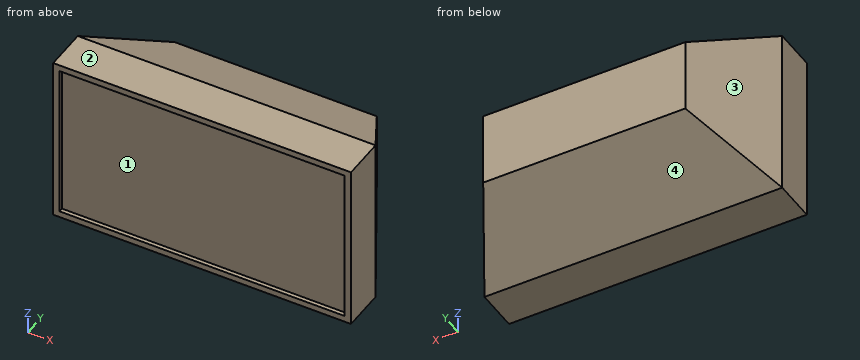
from build123d import *

# Parameters (mm, degrees)
F0_W        = 140
F0_H        = 80
F1_DEPTH    = 60
F2_C1_SIZE2 = 22.5
F2_C1_SIZE  = 40
F2_C2_SIZE2 = 22.5
F2_C2_SIZE  = 40
F2_C3_SIZE2 = 40
F2_C3_SIZE  = 22.5
F2_C4_SIZE2 = 40
F2_C4_SIZE  = 22.5
F3_W        = 134
F3_H        = 74
F4_DEPTH    = 2
F5_DEPTH    = 2


with BuildPart() as f1:
    # F0 (on Front) → F1 (new body)
    with BuildSketch(Plane.XZ):
        Rectangle(F0_W, F0_H)
    extrude(amount=F1_DEPTH)

    # F2: chamfer of 22.5 x 40 on 4 edges, made by hand

    # F2_c1
    f2_c1_edges = [f1.edges().sort_by_distance(p)[0] for p in [
        (0, 0, -40),
    ]]
    f2_c1_side = f1.faces().sort_by_distance((0, -0.45, -40))[0]
    chamfer(f2_c1_edges, length=F2_C1_SIZE, length2=F2_C1_SIZE2, reference=f2_c1_side)

    # F2_c2
    f2_c2_edges = [f1.edges().sort_by_distance(p)[0] for p in [
        (70, 0, 11.25),
    ]]
    f2_c2_side = f1.faces().sort_by_distance((70, -0.45, 11.25))[0]
    chamfer(f2_c2_edges, length=F2_C2_SIZE, length2=F2_C2_SIZE2, reference=f2_c2_side)

    # F2_c3
    f2_c3_edges = [f1.edges().sort_by_distance(p)[0] for p in [
        (-11.25, 0, 40),
    ]]
    f2_c3_side = f1.faces().sort_by_distance((-11.25, 0, 39.55))[0]
    chamfer(f2_c3_edges, length=F2_C3_SIZE, length2=F2_C3_SIZE2, reference=f2_c3_side)

    # F2_c4
    f2_c4_edges = [f1.edges().sort_by_distance(p)[0] for p in [
        (-70, 0, 0),
    ]]
    f2_c4_side = f1.faces().sort_by_distance((-69.55, 0, 0))[0]
    chamfer(f2_c4_edges, length=F2_C4_SIZE, length2=F2_C4_SIZE2, reference=f2_c4_side)

    # F3 (on face) → F4 (join)
    with BuildSketch(Plane.XZ.offset(60)):
        Rectangle(F3_W, F3_H)
    extrude(amount=-F4_DEPTH)

    # F3 (on face) → F5 (cut)
    with BuildSketch(Plane.XZ.offset(60)):
        Rectangle(F3_W, F3_H)
    extrude(amount=-F5_DEPTH, mode=Mode.SUBTRACT)


solid = f1.part
The listing builds one solid part. Answer for the finished solid, in the listing's coordinates (mm). Face numbers are marked on the shaded views. Round coordinates to 2 decimals unless told otherwise and drop trailing zeros. Write each loop counter-clockwise with the first axis right and the second up, starting at its lowest first coordinate (ties: lowest second). Pieces come first, ordered by that corner, then holes. Notation, with made-up numbers: (20, 34.25) - (45, 34.25) arc R20 ccw to (45, 39.25) - close; hole circle Ø3 at (31.5, -5.75). An arc over 180 degrees is marked (long way). Use a Markdown table: item, result. Add a question column.
1. Flat-ended cylindrical pins translate along their axes: P1, Ø6, axis at y = -27.5, z = -3, coming from the -X side; P2, Ø8, axis at x = -42.5, y = -8, coming from the +Z side; P3, Ø12, axis at x = 21.5, y = -17.5, coming from the -Z side. Find the tip coordinate at first contact, or state that the pin passes through.
2. The part is cut by section B-B (x = -5). Write down the section's boundary in (y, z), and give its area (3 significant figures).
3. The part is cut by section D-D (y = -12). Write down the section's boundary in (x, z), and give its area (3 significant figures).
4. For a pull along Z with two mould halves and no side action, classify the marked faces 1, 2, 3 and 4 as +Z half, -Z half, draft (parallel to the pull), parting line (faces both ways), or undercut.
5. The part is cut by section C-C (y = -24). Write down the section's boundary in (x, z).
6. Consider line 1 (Y direction, x = 27.5, z = -16); line 2 (X direction, y = -29, z = -7.5); line 3 (X direction, y = -6.5, z = -7). Determine where each line is inside the solid, lowest interval first.
7. The part is cut by section A-A (z = -2.5). Write down the section's boundary in (x, y).
Reported:
| question | item | result |
|---|---|---|
| 1 | P1 | x = -64.66 |
| 1 | P2 | z = 24.25 |
| 1 | P3 | z = -30.72 |
| 2 | outline | (-60, -40) - (-40, -40) - (0, -17.5) - (0, 17.5) - (-40, 40) - (-60, 40) - (-60, 37) - (-58, 37) - (-58, -37) - (-60, -37) - close |
| 2 | area | 3,750 mm^2 |
| 3 | outline | (-54.25, -24.25) - (54.25, -24.25) - (54.25, 24.25) - (-54.25, 24.25) - close |
| 3 | area | 5,260 mm^2 |
| 4 | face 1 | undercut |
| 4 | face 2 | +Z half |
| 4 | face 3 | draft |
| 4 | face 4 | -Z half |
| 5 | outline | (-61, -31) - (61, -31) - (61, 31) - (-61, 31) - close |
| 6 | line 1 | -58 to 0 |
| 6 | line 2 | -63.81 to 63.81 |
| 6 | line 3 | -51.16 to 51.16 |
| 7 | outline | (-70, -60) - (-67, -60) - (-67, -58) - (67, -58) - (67, -60) - (70, -60) - (70, -40) - (47.5, 0) - (-47.5, 0) - (-70, -40) - close |
